Geometry check sheet. Reference: drawing and pictorial views, mm from the part's lowest x, y, z. A direction names the side the tool comes from. Coordinates: 2 decimals unless noted, no trailing zeros. Order: outer loops, then holes, each group sorted by start corner. A loop starts at its lowest first (then second) coordinate and runs counter-clockwise, first axis right, second up. Notation, with made-up numbers: (-14, -10.5) -> (44, -10.5) arc R19 ccw to (44, 25.5) -> close; hole circle Ø9 at (81, -27). An arc over 180 degrees is marked (long way). Use CSV: the item, a comma, the result in double quotes. Start each with the question number.
1) Sectioned sample at D-D on z = 2.45. Record the boundary of the cut face in (x, y).
2) Release check for a two-part mould opening along Y. For the marked faces 3, 4 and 5 record: released by +Y, released by -Y, zero draft, split by the parting line, or undercut.
3) Go/stop test with flat-tipped pins: pin 1 (2 mm diameter, centred on x = 3, z = 5, fed in from +Y); pin 2 (1.8 mm diameter, centred on x = 8.55, y = 18.45, fed in from -Z); pin 3 (2 mm diameter, centred on y = 15, z = 2.5, fed in from -X); pin 4 (1 mm diameter, centred on x = 11, z = 2.5, fed in from +Y). Record where each tip stops, or that it passes through.
4) Sectioned sample at A-A on y = 13.5. Record the boundary of the cut face in (x, z) (1 decimal).
5) Tool access check on the marked faces 1 and 2. Record the directions out of +Z, -Z, +X, -X, +Y, -Y that give a thin tool (end or side, any length) a straight path to the whole face; none if there is none.
6) Sectioned sample at C-C on x = 4. Record the boundary of the cut face in (y, z).
7) Sectioned sample at B-B on z = 0.9. Give the number of separate pieces and of enclosed holes in the cut face, then the cut area to 3 significant figures.
8) Scan lines: line 1 along X through (y, z) = (8.5, 3.95); line 2 along Y through (x, z) = (8, 4.3) (1 decimal). Record each from-to range of solid material in increasing order.
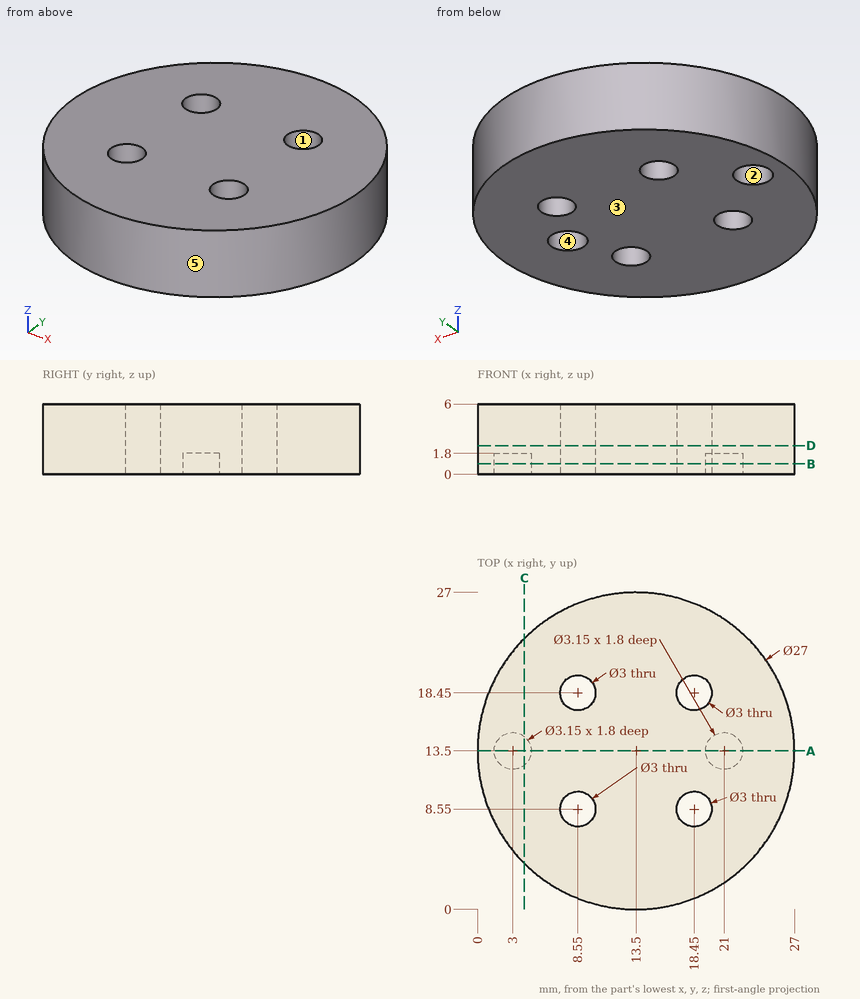
Answers follow:
1,outline,"circle Ø27 at (13.5, 13.5); hole circle Ø3 at (8.55, 8.55); hole circle Ø3 at (8.55, 18.45); hole circle Ø3 at (18.45, 8.55); hole circle Ø3 at (18.45, 18.45)"
2,face 3,"zero draft"
2,face 4,"undercut"
2,face 5,"split by the parting line"
3,pin 1,"stops at y = 23.09"
3,pin 2,"passes through"
3,pin 3,"stops at x = 0.01"
3,pin 4,"stops at y = 26.85"
4,outline,"(0, 0) -> (1.4, 0) -> (1.4, 1.8) -> (4.6, 1.8) -> (4.6, 0) -> (19.4, 0) -> (19.4, 1.8) -> (22.6, 1.8) -> (22.6, 0) -> (27, 0) -> (27, 6) -> (0, 6) -> close"
5,face 1,"+Z, -Z"
5,face 2,"-Z"
6,outline,"(3.91, 0) -> (12.28, 0) -> (12.28, 1.8) -> (14.72, 1.8) -> (14.72, 0) -> (23.09, 0) -> (23.09, 6) -> (3.91, 6) -> close"
7,separate pieces,"1"
7,enclosed holes,"6"
7,area,"529 mm²"
8,line 1,"x = 0.96 to 7.05, 10.05 to 16.95, 19.95 to 26.04"
8,line 2,"y = 1.2 to 7.2, 9.9 to 17.1, 19.8 to 25.8"
